```python
from build123d import *

# Parameters (mm, degrees)
F1_DEPTH  = 2.54
F3_DEPTH  = 12.7
F5_DEPTH  = 52.071
F7_DEPTH  = 76.2
F9_DEPTH  = 25.4
F10_W     = 50.673
F10_H     = 12.954
F10_W_2   = 12.954
F10_H_2   = 37.973
F11_DEPTH = 0.635
F12_DEPTH = 13.462
F14_DEPTH = 1.905
F15_R     = 4.7625
F15_R_2   = 3.175
F16_DEPTH = 25.4
F17_R     = 1.2763153823
F17_R_2   = 1.27
F18_DEPTH = 25.4


# Not quite as in the source:
# - ends of sketch curves that miss each other by under 0.0002 mm in the source are joined


with BuildPart() as f1:
    # F0 (on Front) → F1 (new body)
    with BuildSketch(Plane.XZ):
        with BuildLine():
            Line((30.48, 31.75), (-30.48, 31.75))
            ThreePointArc((-30.48, 31.75), (-44.8484097937, 25.7984097937), (-50.8, 11.43))
            Line((-50.8, 11.43), (-50.8, -11.43))
            ThreePointArc((-50.8, -11.43), (-44.8484097937, -25.7984097937), (-30.48, -31.75))
            Line((-30.48, -31.75), (30.48, -31.75))
            ThreePointArc((30.48, -31.75), (44.8484097937, -25.7984097937), (50.8, -11.43))
            Line((50.8, -11.43), (50.8, 11.43))
            ThreePointArc((50.8, 11.43), (44.8484097937, 25.7984097937), (30.48, 31.75))
        make_face()
    extrude(amount=F1_DEPTH)

    # F2 (on Front) → F3 (join)
    with BuildSketch(Plane.XZ):
        with BuildLine():
            ThreePointArc((33.02, 0), (27.0684097937, 14.3684097937), (12.7, 20.32))
            Line((12.7, 20.32), (-12.7, 20.32))
            ThreePointArc((-12.7, 20.32), (-27.0684097937, 14.3684097937), (-33.02, 0))
            ThreePointArc((-33.02, 0), (-27.0684097937, -14.3684097937), (-12.7, -20.32))
            Line((-12.7, -20.32), (12.7, -20.32))
            ThreePointArc((12.7, -20.32), (27.0684097937, -14.3684097937), (33.02, 0))
        make_face()
        with BuildLine():
            ThreePointArc((-30.48, 0), (-25.2723585695, 12.5723585695), (-12.7, 17.78))
            Line((-12.7, 17.78), (12.7, 17.78))
            ThreePointArc((12.7, 17.78), (25.2723585695, 12.5723585695), (30.48, 0))
            ThreePointArc((30.48, 0), (25.2723585695, -12.5723585695), (12.7, -17.78))
            Line((12.7, -17.78), (-12.7, -17.78))
            ThreePointArc((-12.7, -17.78), (-25.2723585695, -12.5723585695), (-30.48, 0))
        make_face(mode=Mode.SUBTRACT)
    extrude(amount=-F3_DEPTH)

    # F4 (on face) → F5 (cut, through all)
    with BuildSketch(Plane.XY.offset(20.32)):
        Polygon((6.604, 12.7), (0, 12.7), (-6.604, 12.7), (-6.604, 0), (6.604, 0), align=None)
    extrude(amount=-F5_DEPTH, mode=Mode.SUBTRACT)

    # F6 (on Right) → F7 (cut, symmetric)
    with BuildSketch(Plane.YZ):
        Polygon((0, 6.604), (0, 0), (0, -6.604), (12.7, -6.604), (12.7, 6.604), align=None)
    extrude(amount=F7_DEPTH, both=True, mode=Mode.SUBTRACT)

    # F8 (on face) → F9 (cut)
    with BuildSketch(Plane(origin=(0, 0, 0), x_dir=(-1, 0, 0), z_dir=(0, 1, 0))):
        with BuildLine():
            Line((12.7, 15.875), (-12.7, 15.875))
            ThreePointArc((-12.7, 15.875), (-23.9253201513, 11.2253201513), (-28.575, 0))
            ThreePointArc((-28.575, 0), (-23.9253201513, -11.2253201513), (-12.7, -15.875))
            Line((-12.7, -15.875), (12.7, -15.875))
            ThreePointArc((12.7, -15.875), (23.9253201513, -11.2253201513), (28.575, 0))
            ThreePointArc((28.575, 0), (23.9253201513, 11.2253201513), (12.7, 15.875))
        make_face()
    extrude(amount=-F9_DEPTH, mode=Mode.SUBTRACT)

    # F10 (on face) → F11 (cut)
    with BuildSketch(Plane(origin=(0, 0, 0), x_dir=(-1, 0, 0), z_dir=(0, 1, 0))):
        with Locations((-31.8135, 0)):
            Rectangle(F10_W, F10_H)
        with Locations((0, 25.4635)):
            Rectangle(F10_W_2, F10_H_2)
        Rectangle(F10_W_2, F10_H)
        with Locations((31.8135, 0)):
            Rectangle(F10_W, F10_H)
        with Locations((0, -25.4635)):
            Rectangle(F10_W_2, F10_H_2)
    extrude(amount=-F11_DEPTH, mode=Mode.SUBTRACT)

    # F12 (cut): faces of the model
    f12_faces = [f1.faces().sort_by_distance(p)[0] for p in [
        (9.652, 12.7, -20.0320986266),
        (30.5624774214, 12.7, 6.8919013734),
        (-30.5624774214, 12.7, -6.8919013734),
        (-6.8919013734, 12.7, 19.05),
    ]]
    extrude(f12_faces, amount=-F12_DEPTH, mode=Mode.SUBTRACT)

    # F13 (on face) → F14 (join)
    with BuildSketch(Plane.XZ.offset(2.54)):
        with BuildLine():
            Line((-12.7, -15.875), (12.7, -15.875))
            ThreePointArc((12.7, -15.875), (23.9253201513, -11.2253201513), (28.575, 0))
            ThreePointArc((28.575, 0), (23.9253201513, 11.2253201513), (12.7, 15.875))
            Line((12.7, 15.875), (-12.7, 15.875))
            ThreePointArc((-12.7, 15.875), (-23.9253201513, 11.2253201513), (-28.575, 0))
            ThreePointArc((-28.575, 0), (-23.9253201513, -11.2253201513), (-12.7, -15.875))
        make_face()
    extrude(amount=-F14_DEPTH)

    # F15 (on face) → F16 (cut)
    with BuildSketch(Plane(origin=(0, -0.635, 0), x_dir=(-1, 0, 0), z_dir=(0, 1, 0))):
        Circle(F15_R)
        with Locations((-25.4, 0)):
            Circle(F15_R_2)
        with Locations((25.4, 0)):
            Circle(F15_R_2)
    extrude(amount=-F16_DEPTH, mode=Mode.SUBTRACT)

    # F17 (on face) → F18 (cut)
    with BuildSketch(Plane(origin=(0, 0, 0), x_dir=(-1, 0, 0), z_dir=(0, 1, 0))):
        Polygon((47.6680542115, -27.4815886288), (51.1667876586, -29.4946501669), (47.6696745814, -27.4787697193), align=None)
        with BuildLine():
            Line((47.0404791933, -28.5733623005), (47.6680542115, -27.4815886288))
            Line((47.6680542115, -27.4815886288), (47.6696745814, -27.4787697193))
            Line((47.6696745814, -27.4787697193), (48.3063004883, -26.3712504847))
            Line((48.3063004883, -26.3712504847), (43.0570225864, -23.3538525016))
            ThreePointArc((43.0570225864, -23.3538525016), (41.2580877478, -23.7846525937), (41.7912012914, -25.5559643173))
            Line((41.7912012914, -25.5559643173), (47.0404791933, -28.5733623005))
        make_face()
        with Locations((-25.1277598759, -14.4543864422)):
            Circle(F17_R)
        with Locations((-25.1438466209, 14.4120964147)):
            Circle(F17_R_2)
        with Locations((25.1215984181, 14.4508421512)):
            Circle(F17_R_2)
        with Locations((25.0963969645, -14.4945646834)):
            Circle(F17_R_2)
        with BuildLine():
            ThreePointArc((-41.8649914427, -25.5417502167), (-41.2719571065, -23.8052669732), (-43.0327445767, -23.2888453782))
            Line((-43.0327445767, -23.2888453782), (-48.1358024341, -26.2243068229))
            Line((-48.1358024341, -26.2243068229), (-46.8692956724, -28.4260244757))
            Line((-46.8692956724, -28.4260244757), (-41.8629335005, -25.5461858486))
            Line((-41.8629335005, -25.5461858486), (-41.8649914427, -25.5417502167))
        make_face()
        with BuildLine():
            ThreePointArc((-43.0465700311, 23.2475518967), (-41.3065716807, 23.7045275153), (-41.7691664779, 25.443040394))
            Line((-41.7691664779, 25.443040394), (-41.7793320219, 25.4488488271))
            Line((-41.7793320219, 25.4488488271), (-42.2095022754, 25.6963553049))
            Line((-42.2095022754, 25.6963553049), (-46.0359033246, 27.8979465087))
            Line((-46.0359033246, 27.8979465087), (-47.302629882, 25.6963553049))
            Line((-47.302629882, 25.6963553049), (-43.0465700311, 23.2475518967))
        make_face()
        with BuildLine():
            Line((46.6254135383, 28.2857347472), (41.7498114349, 25.4811139895))
            ThreePointArc((41.7498114349, 25.4811139895), (41.2839564144, 23.7439684966), (43.0223799296, 23.2829055446))
            Line((43.0223799296, 23.2829055446), (47.8919203, 26.0840170944))
            Line((47.8919203, 26.0840170944), (46.6254135383, 28.2857347472))
        make_face()
    extrude(amount=-F18_DEPTH, mode=Mode.SUBTRACT)


solid = f1.part
```
CAD build for the part. Positions are in the model's coordinates, mm. A direction names the side the tool comes from. Coordinates: 2 decimals unless noted, no trailing zeros. Loops run counter-clockwise (first coordinate to the right, second up) from the corner with the lowest first, then second, coordinate; pieces in that order, holes last. Notation, with made-up numbers: (7, 82) - (11, 82) arc R17 cw to (11, 94) - close; hole circle Ø8 at (29.25, 33). An arc over 180 degrees is marked (long way). Use CSV: the item, a comma, the result in double quotes. Start each with the question number.
Q1. Cut at B-B, the plane z = 0. List the corners of the cut face in (x, y) (1 decimal), then the cut area to 3 significant figures.
Q2. Two-plate mould, pull along X, no slides. Class faces 1 (the cylindrical face through (37.76, -1.25, 30.4)), 2 (the cylindrical face through (-49.457, -1.252, 18.695)), 3 (the cylindrical face through (-24.96, -1.53, 15.71)): +X half, -X half, draft (parallel to the pull), parting line (faces both ways), or undercut.
Q3. Probe probe 1 along Z at (x, y) = (0, -1.9); probe 2 along X at (y, z) = (-2.1, -1); probe 3 along X at (y, z) = (-0.75, 24). List the from-to ranges inside material, lowest first. Write a range as from..to.
Q4. Cut at C-C, the plane x = 39.5. List the corners of the cut face in (y, z) (3 decimals), then the cut area to 3 significant figures.
Q5. 3-axis set-ups, long thin cutter, end or side, ignore diameter. For faces 4 (the cylindrical face through (-49.522, -1.252, -18.524)), 5 (the flat face through (-20.3, -0.762, -16.5)), 6 (the flat face through (44.427, -1.252, 24.042)), 7 (the flat face through (-42.804, -1.252, -26.138)): which of +Z, -Z, +X, -X, +Y, -Y reach the whole face in a straight line?
Q6. Drop flat-ended pins along their axis: P1, Ø2, axis at x = -25.12, z = 14.45, coming from the +Y side; P2, Ø0.5, axis at y = -0.5, z = -26, coming from the -X side; P3, Ø0.5, axis at x = -37, y = 0, coming from the +Z side. Give the stop position or say it passes through.
Here are the results:
1,outline,"(-50.8, -2.5) - (-28.6, -2.5) - (-28.6, -0.6) - (-50.8, -0.6) - close; (-22.2, -2.5) - (-4.8, -2.5) - (-4.8, -0.6) - (-22.2, -0.6) - close; (4.8, -2.5) - (22.2, -2.5) - (22.2, -0.6) - (4.8, -0.6) - close; (28.6, -2.5) - (50.8, -2.5) - (50.8, -0.6) - (28.6, -0.6) - close"
1,area,"151 mm2"
2,face 1,"+X half"
2,face 2,"-X half"
2,face 3,"undercut"
3,probe 1,"-31.75..-4.76, 4.76..31.75"
3,probe 2,"-50.8..-28.41, -22.39..-4.66, 4.66..22.39, 28.41..50.8"
3,probe 3,"-46.45..-44.27, -41.17..41.18, 44.35..46.45"
4,outline,"(-2.54, -29.638) - (0, -29.638) - (0, -6.477) - (-0.635, -6.477) - (-0.635, 6.477) - (0, 6.477) - (0, 29.638) - (-2.54, 29.638) - close"
4,area,"142 mm2"
5,face 4,"-Z, -X, +Y, -Y"
5,face 5,"+Y"
5,face 6,"+Y, -Y"
5,face 7,"-X, +Y, -Y"
6,P1,"through"
6,P2,"x = -43"
6,P3,"z = 30.76"
